Read the model definition and answer for the solid it produces. Units are mm, in the model's axes. Face numbers are marked on the shaded views. A direction names the side the tool comes from. Round coordinates to 2 decimals unless told otherwise and drop trailing zeros. Write each loop counter-clockwise with the first axis right and the second up, starting at its lowest first coordinate (ties: lowest second). Pieces come first, ordered by that corner, then holes. Notation, with made-up numbers: (60.25, 77) - (110.25, 77) arc R7 cw to (110.25, 87) - close; hole circle Ø2 at (23.5, 78.25). An arc over 180 degrees is marked (long way). One line per item, written item: value. Start each with the question number.
(1) The mould has two halves that part along Y. Classify the marked faces 4, 5 and 6: +Y half, -Y half, draft (parallel to the pull), parting line (faces both ways), or undercut.
(2) Find the intervals of material crossed by L1, parallel to Y at x = 0, z = 32; L2, parallel to Z at x = 14.5, y = -11.5, in increasing order.
(3) Flat-ended cylindrical pins translate along their axes: pin 1 Ø8 at (x, z) = (-21.5, 24.5) entering from +Y; pin 2 Ø8 at (x, z) = (23, 36) entering from +Y; pin 3 Ø4 at (y, z) = (-11.5, 48.5) entering from -X. Find the tip coordinate at first contact, or state that the pin passes through.
(4) A cutting plane is placed at C-C, the plane x = -13. Determine the outline of the cut face in (y, z), plus the area to 3 significant figures.
(5) For the marked faces 1, 2 and 3, determine the directions among +Z, -Z, +X, -X, +Y, -Y from which every point of the face is accessible in a straight line to the end or side of a thin tool.
(6) A cutting plane is placed at A-A, the plane z = 4.5. Determine the outline of the cut face in (x, y) (1 decimal), plus the area to 3 significant figures.
(7) A cutting plane is placed at D-D, the plane y = 41.5. Determine the outline of the cut face in (x, z), plus the area to 3 significant figures.
(8) A cutting plane is placed at B-B, the plane y = 0. Determine the outline of the cut face in (x, z), plus the area to 3 significant figures.
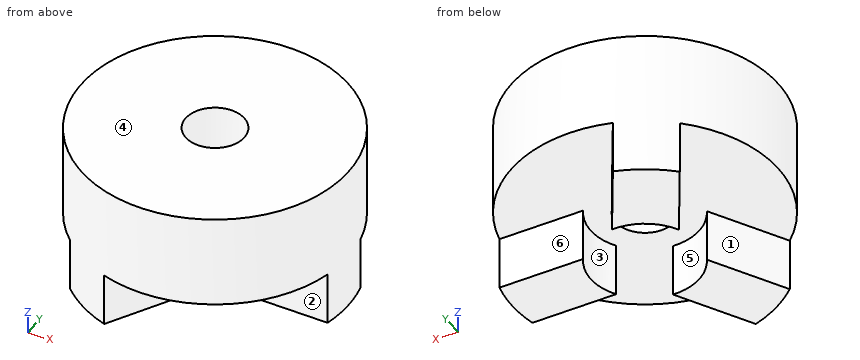
from build123d import *

# Parameters (mm, degrees)
SKETCH1_R           = 50
SKETCH1_R_2         = 11
BOSS_EXTRUDE1_DEPTH = 55
CUT_EXTRUDE2_DEPTH  = 20


with BuildPart() as part:
    # Sketch1 → Boss-Extrude1 (new body)
    with BuildSketch(Plane.XY):
        Circle(SKETCH1_R)
        Circle(SKETCH1_R_2, mode=Mode.SUBTRACT)
    extrude(amount=BOSS_EXTRUDE1_DEPTH)

    # Sketch3 → Cut-Extrude2 (cut)
    with BuildSketch(Plane(origin=(0, 0, 0), x_dir=(-1, 0, 0), z_dir=(0, 0, -1))):
        with BuildLine():
            Line((-48.774993593, -11), (-17.145475472, -11))
            ThreePointArc((-17.145475472, -11), (-20.370746897, 0), (-17.145475472, 11))
            Line((-17.145475472, 11), (-48.774993593, 11))
            ThreePointArc((-48.774993593, 11), (-25, 43.301270189), (14.861217355, 47.740383521))
            Line((14.861217355, 47.740383521), (-0.953541706, 20.348417319))
            ThreePointArc((-0.953541706, 20.348417319), (10.185373449, 17.641584307), (18.099017178, 9.348417319))
            Line((18.099017178, 9.348417319), (33.913776238, 36.740383521))
            ThreePointArc((33.913776238, 36.740383521), (50, 0), (33.913776238, -36.740383521))
            Line((33.913776238, -36.740383521), (18.099017178, -9.348417319))
            ThreePointArc((18.099017178, -9.348417319), (10.185373449, -17.641584307), (-0.953541706, -20.348417319))
            Line((-0.953541706, -20.348417319), (14.861217355, -47.740383521))
            ThreePointArc((14.861217355, -47.740383521), (-25, -43.301270189), (-48.774993593, -11))
        make_face()
    extrude(amount=-CUT_EXTRUDE2_DEPTH, mode=Mode.SUBTRACT)


solid = part.part
Here are the results:
1. face 4: draft
1. face 5: undercut
1. face 6: +Y half
2. L1: -50 to -11, 11 to 50
2. L2: 20 to 55
3. pin 1: y = 46.84
3. pin 2: y = 46.25
3. pin 3: x = -49.09
4. outline: (-48.28, 20) - (-44.52, 20) - (-44.52, 0) - (-15.68, 0) - (-15.68, 20) - (15.68, 20) - (15.68, 0) - (44.52, 0) - (44.52, 20) - (48.28, 20) - (48.28, 55) - (-48.28, 55) - close
4. area: 4,530 mm²
5. face 1: -Z, -X
5. face 2: -Z, +X, -Y
5. face 3: -Z
6. outline: (-33.9, -36.7) arc R50 ccw to (-14.9, -47.7) - (1, -20.3) arc R20.4 cw to (-18.1, -9.3) - close; (-33.9, 36.7) - (-18.1, 9.3) arc R20.4 cw to (1, 20.3) - (-14.9, 47.7) arc R50 ccw to start; (17.1, -11) - (48.8, -11) arc R50 ccw to (48.8, 11) - (17.1, 11) arc R20.4 cw to start
6. area: 2,000 mm²
7. outline: (-27.89, 0) - (-11.26, 0) - (-11.26, 20) - (27.89, 20) - (27.89, 55) - (-27.89, 55) - close
7. area: 2,280 mm²
8. outline: (-50, 20) - (-11, 20) - (-11, 55) - (-50, 55) - close; (11, 20) - (20.37, 20) - (20.37, 0) - (50, 0) - (50, 55) - (11, 55) - close
8. area: 3,320 mm²
